The model under review builds one solid part; all positions refer to its coordinate system, in mm. Face numbers are marked on the shaded views. A direction names the side the tool comes from. Give positions to 0.01 mm unless a question says otherwise; leave off trailing zeros. Order: outer loops, then holes, each group sorted by start corner. A loop starts at its lowest first (then second) coordinate and runs counter-clockwise, first axis right, second up. Notation, with made-up numbers: (32.25, -36) - (88.25, -36) arc R31 ccw to (88.25, -7) - close; hole circle Ø1 at (30, -35). An arc over 180 degrees is marked (long way). Put each result on its own line as item: value.
```python
from build123d import *

# Parameters (mm, degrees)
SKETCH1_W           = 100
SKETCH1_H           = 120
BOSS_EXTRUDE1_DEPTH = 20
SKETCH2_W           = 19.05
SKETCH2_H           = 19.05
CUT_EXTRUDE1_DEPTH  = 20
SKETCH3_R           = 1.5
CUT_EXTRUDE2_DEPTH  = 20
SKETCH5_R           = 5
SKETCH5_R_2         = 2.65
CUT_EXTRUDE3_DEPTH  = 21
SKETCH6_W           = 60
SKETCH6_H           = 30
CUT_EXTRUDE4_DEPTH  = 10
CUT_EXTRUDE5_DEPTH  = 21
SKETCH8_W           = 71
SKETCH8_H           = 70.95
CUT_EXTRUDE6_DEPTH  = 21
CHAMFER1_SIZE       = 10
SKETCH9_W           = 50
SKETCH9_H           = 10
SKETCH9_W_2         = 40
SKETCH9_H_2         = 30
CUT_EXTRUDE7_DEPTH  = 21
CHAMFER2_SIZE       = 5
CUT_EXTRUDE8_DEPTH  = 21
SKETCH12_W          = 80
SKETCH12_H          = 5
CUT_EXTRUDE9_DEPTH  = 21


with BuildPart() as part:
    # Sketch1 → Boss-Extrude1 (new body)
    with BuildSketch(Plane(origin=(0, 0, 0), x_dir=(0, 0, -1), z_dir=(1, 0, 0))):
        with Locations((-50, 60)):
            Rectangle(SKETCH1_W, SKETCH1_H)
    boss_extrude1 = extrude(amount=BOSS_EXTRUDE1_DEPTH)

    # Sketch2 → Cut-Extrude1 (cut)
    with BuildSketch(Plane(origin=(20, 0, 0), x_dir=(0, 0, -1), z_dir=(1, 0, 0))):
        with Locations((-80.475, 29.525)):
            Rectangle(SKETCH2_W, SKETCH2_H)
    cut_extrude1 = extrude(amount=-CUT_EXTRUDE1_DEPTH, mode=Mode.SUBTRACT)

    # Sketch3 → Cut-Extrude2 (cut)
    with BuildSketch(Plane.XY.offset(100)):
        with Locations((10, 34.605)):
            Circle(SKETCH3_R)
        with Locations((10, 24.445)):
            Circle(SKETCH3_R)
    cut_extrude2 = extrude(amount=-CUT_EXTRUDE2_DEPTH, mode=Mode.SUBTRACT)

    # Mirror1: Boss-Extrude1, Cut-Extrude1, Cut-Extrude2 across plane
    add(boss_extrude1.mirror(Plane(origin=(20, 0, 0), x_dir=(1, 0, 0), z_dir=(0, 0, 1))))
    add(cut_extrude1.mirror(Plane(origin=(20, 0, 0), x_dir=(1, 0, 0), z_dir=(0, 0, 1))), mode=Mode.SUBTRACT)
    add(cut_extrude2.mirror(Plane(origin=(20, 0, 0), x_dir=(1, 0, 0), z_dir=(0, 0, 1))), mode=Mode.SUBTRACT)

    # Sketch5 → Cut-Extrude3 (cut, through all)
    with BuildSketch(Plane(origin=(20, 0, 0), x_dir=(0, 0, -1), z_dir=(1, 0, 0))):
        with Locations((0, 25.5)):
            Circle(SKETCH5_R)
        with Locations((-18.5, 25.5)):
            Circle(SKETCH5_R_2)
        with Locations((18.5, 25.5)):
            Circle(SKETCH5_R_2)
    extrude(amount=-CUT_EXTRUDE3_DEPTH, mode=Mode.SUBTRACT)

    # Sketch6 → Cut-Extrude4 (cut)
    with BuildSketch(Plane(origin=(20, 0, 0), x_dir=(0, 0, -1), z_dir=(1, 0, 0))):
        with Locations((0, 25.5)):
            Rectangle(SKETCH6_W, SKETCH6_H)
    extrude(amount=-CUT_EXTRUDE4_DEPTH, mode=Mode.SUBTRACT)

    # Sketch7 → Cut-Extrude5 (cut, through all)
    with BuildSketch(Plane(origin=(20, 0, 0), x_dir=(0, 0, -1), z_dir=(1, 0, 0))):
        with BuildLine():
            Line((5, 109.05), (5, 89.05))
            ThreePointArc((5, 89.05), (0, 84.05), (-5, 89.05))
            Line((-5, 89.05), (-5, 109.05))
            ThreePointArc((-5, 109.05), (0, 114.05), (5, 109.05))
        make_face()
        with BuildLine():
            Line((-16, 109.05), (-16, 89.05))
            ThreePointArc((-16, 89.05), (-18.5, 86.55), (-21, 89.05))
            Line((-21, 89.05), (-21, 109.05))
            ThreePointArc((-21, 109.05), (-18.5, 111.55), (-16, 109.05))
        make_face()
        with BuildLine():
            Line((16, 109.05), (16, 89.05))
            ThreePointArc((16, 89.05), (18.5, 86.55), (21, 89.05))
            Line((21, 89.05), (21, 109.05))
            ThreePointArc((21, 109.05), (18.5, 111.55), (16, 109.05))
        make_face()
    extrude(amount=-CUT_EXTRUDE5_DEPTH, mode=Mode.SUBTRACT)

    # Sketch8 → Cut-Extrude6 (cut, through all)
    with BuildSketch(Plane(origin=(20, 0, 0), x_dir=(0, 0, -1), z_dir=(1, 0, 0))):
        with Locations((-64.5, 84.525)):
            Rectangle(SKETCH8_W, SKETCH8_H)
        with Locations((64.5, 84.525)):
            Rectangle(SKETCH8_W, SKETCH8_H)
    extrude(amount=-CUT_EXTRUDE6_DEPTH, mode=Mode.SUBTRACT)

    # Chamfer1
    chamfer1_edges = [part.edges().sort_by_distance(p)[0] for p in [
        (10, 49.05, 100),
        (10, 120, 29),
        (10, 49.05, 29),
        (10, 120, -29),
        (10, 49.05, -100),
        (10, 49.05, -29),
    ]]
    chamfer(chamfer1_edges, length=CHAMFER1_SIZE)

    # Sketch9 → Cut-Extrude7 (cut, through all)
    with BuildSketch(Plane(origin=(20, 0, 0), x_dir=(0, 0, -1), z_dir=(1, 0, 0))):
        with Locations((-65, 5)):
            Rectangle(SKETCH9_W, SKETCH9_H)
        with Locations((65, 5)):
            Rectangle(SKETCH9_W, SKETCH9_H)
        with Locations((0, 64.05)):
            Rectangle(SKETCH9_W_2, SKETCH9_H_2)
    extrude(amount=-CUT_EXTRUDE7_DEPTH, mode=Mode.SUBTRACT)

    # Chamfer2
    chamfer2_edges = [part.edges().sort_by_distance(p)[0] for p in [
        (10, 10, 90),
        (10, 10, 40),
        (10, 10, -40),
        (10, 10, -90),
        (10, 49.05, 20),
        (10, 79.05, 20),
        (10, 79.05, -20),
        (10, 49.05, -20),
        (15, 10.5, 30),
        (15, 40.5, 30),
        (15, 40.5, -30),
        (15, 10.5, -30),
    ]]
    chamfer(chamfer2_edges, length=CHAMFER2_SIZE)

    # Sketch11 → Cut-Extrude8 (cut, through all)
    with BuildSketch(Plane(origin=(20, 0, 0), x_dir=(0, 0, -1), z_dir=(1, 0, 0))):
        Polygon((-40, 25.5), (-45.5, 20), (-40, 20), align=None)
        Polygon((-49, 39.05), (-60.95, 27.1), (-60.95, 39.05), align=None)
    cut_extrude8 = extrude(amount=-CUT_EXTRUDE8_DEPTH, mode=Mode.SUBTRACT)

    # Mirror2: Cut-Extrude8 across plane
    add(cut_extrude8.mirror(Plane.XY), mode=Mode.SUBTRACT)

    # Sketch12 → Cut-Extrude9 (cut, through all)
    with BuildSketch(Plane.ZY):
        with Locations((0, 2.5)):
            Rectangle(SKETCH12_W, SKETCH12_H)
    extrude(amount=-CUT_EXTRUDE9_DEPTH, mode=Mode.SUBTRACT)


solid = part.part
```
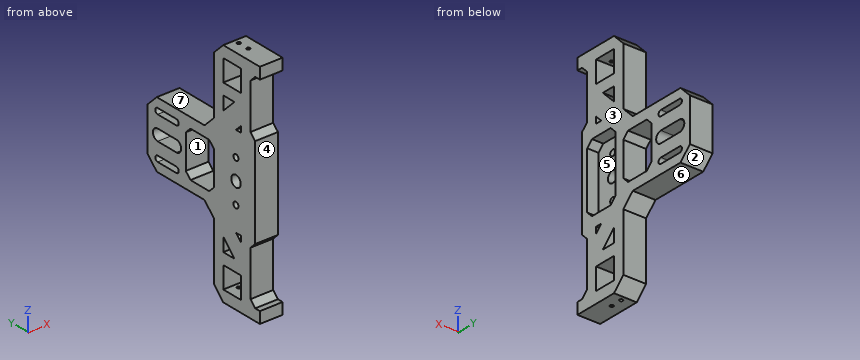
(1) Wall thickness on L1, parallel to Y at x = 15.5, z = 9.5; L2, parallel to Z at x = 4.5, y = 93; L3, parallel to Y at x = 10, z = 97 (3 decimals): over which ranges is each line inside the solid? List them lowest first.
The answers:
L1: 5 to 10.5, 40.5 to 49.05, 79.05 to 120
L2: -29 to -21, -16 to -5, 5 to 16, 21 to 29
L3: 0 to 22.945, 25.945 to 33.105, 36.105 to 42.05
(2) Take a section at B-B, the plane y = 103.5. Write out the cut boundary in (x, z).
The answers:
outline: (0, -29) - (20, -29) - (20, -21) - (0, -21) - close; (0, -16) - (20, -16) - (20, -5) - (0, -5) - close; (0, 5) - (20, 5) - (20, 16) - (0, 16) - close; (0, 21) - (20, 21) - (20, 29) - (0, 29) - close
(3) Take a section at D-D, the plane x = 17. Count the separate pieces of the cut face and the enclosed holes in it, then the cut area to 3 significant figures.
The answers:
separate pieces: 1
enclosed holes: 11
area: 8,160 mm^2
(4) Clearance check with flat-ended pins moving along their axes: pin 1 Ø1.5 at (x, y) = (11.5, 92) entering from -Z; pin 2 Ø12 at (x, z) = (8.5, -32) entering from +Y; pin 3 Ø10 at (x, y) = (11.5, 68) entering from +Z. State where each tip first meets the part, or that it passes through.
The answers:
pin 1: z = -29
pin 2: y = 113
pin 3: z = 29
(5) Take a section at A-A, the plane z = 0. Write out the cut boundary in (x, y).
The answers:
outline: (0, 5) - (20, 5) - (20, 10.5) - (10, 10.5) - (10, 20.5) - (0, 20.5) - close; (0, 30.5) - (10, 30.5) - (10, 40.5) - (20, 40.5) - (20, 49.05) - (0, 49.05) - close; (0, 79.05) - (20, 79.05) - (20, 84.05) - (0, 84.05) - close; (0, 114.05) - (20, 114.05) - (20, 120) - (0, 120) - close
(6) For the marked faces 4, 5, 6 and 7, list the 3-axis set-ups (+Z, -Z, +X, -X, +Y, -Y) from which the entire face can be reached by the end or side of a thin tool; tool diameter is ignored.
The answers:
face 4: +X, -X, -Y
face 5: +X
face 6: -Z, +X, -X, +Y
face 7: +Z, +X, -X, +Y
(7) Take a section at C-C, the plane z = 79. Write out the cut boundary in (x, y), then the cut area to 3 significant figures.
The answers:
outline: (0, 10) - (20, 10) - (20, 20) - (0, 20) - close; (0, 39.05) - (20, 39.05) - (20, 49.05) - (0, 49.05) - close
area: 400 mm^2
(8) The part is to be moulded in two halves that separate along Y. For the marked faces 1, 2 and 3, say which applies: pulls with the +Y half, pulls with the -Y half, needs draft (parallel to the pull), parting line crosses it, or undercut.
The answers:
face 1: undercut
face 2: pulls with the +Y half
face 3: needs draft
